Here's how the part is built. I have some questions about the finished solid (model axes, mm). Give positions to 0.01 mm unless a question says otherwise; leave off trailing zeros. Loops run counter-clockwise (first coordinate to the right, second up) from the corner with the lowest first, then second, coordinate; pieces in that order, holes last. Notation, with made-up numbers: (-40, -34) -> (9, -34) arc R27 cw to (9, -5) -> close; hole circle Ø9 at (19.5, 77.25). An arc over 180 degrees is marked (long way). Answer in a Markdown table with one row per item. Add a question column.
Item 1: If we section it at A-A (y = 663): Write out the boundary of the cut face in (x, z).
Item 2: If I drill on line 1 (X direction, y = 740.5, z = -6); line 2 (X direction, y = 880, z = 0); line 3 (X direction, y = 1176, z = 1), over which ranges is the centre line in solid material (lowest first)?
Item 3: For P1, Ø3, axis at x = 0.5, y = 414.5, coming from the -Z side; P2, Ø5, axis at y = 936, z = -1.5, coming from the +X side; P3, Ø8, axis at y = 772.5, z = -0.5, coming from the -X side; P4, Ø5.5, axis at x = 0, z = 0, coming from the -Y side, each with a flat end and sliding along its axis, tell me the tip position at first contact or that it passes through.
```python
from build123d import *

# Parameters (mm, degrees)
BOSS_EXTRU_2_DEPTH      = 1300
ESQUISSE5_R             = 3
ENL_V_MAT_EXTRU_1_DEPTH = 1301.389364767


with BuildPart() as part:
    # Esquisse4 → Boss.-Extru.2 (new body)
    with BuildSketch(Plane(origin=(0, 0, 0), x_dir=(1, 0, 0), z_dir=(0, 1, 0))):
        with BuildLine():
            Line((-17.5, 22.5), (-5, 22.5))
            ThreePointArc((-5, 22.5), (-7.5, 20), (-5, 17.5))
            Line((-5, 17.5), (5, 17.5))
            ThreePointArc((5, 17.5), (7.5, 20), (5, 22.5))
            Line((5, 22.5), (17.5, 22.5))
            ThreePointArc((17.5, 22.5), (21.035534799, 21.035533013), (22.5, 17.499997475))
            Line((22.5, 17.499997475), (22.5, 4.999997475))
            ThreePointArc((22.5, 4.999997475), (20, 7.499997475), (17.5, 4.999997475))
            Line((17.5, 4.999997475), (17.5, -5.000002525))
            ThreePointArc((17.5, -5.000002525), (20, -7.500002525), (22.5, -5.000002525))
            Line((22.5, -5.000002525), (22.5, -17.500002525))
            ThreePointArc((22.5, -17.500002525), (21.035533013, -21.035534799), (17.5, -22.5))
            Line((17.5, -22.5), (5, -22.5))
            ThreePointArc((5, -22.5), (7.5, -20), (5, -17.5))
            Line((5, -17.5), (-5, -17.5))
            ThreePointArc((-5, -17.5), (-7.5, -20), (-5, -22.5))
            Line((-5, -22.5), (-17.5, -22.5))
            ThreePointArc((-17.5, -22.5), (-21.035533906, -21.035533906), (-22.5, -17.5))
            Line((-22.5, -17.5), (-22.5, -5))
            ThreePointArc((-22.5, -5), (-20, -7.5), (-17.5, -5))
            Line((-17.5, -5), (-17.5, 5))
            ThreePointArc((-17.5, 5), (-20, 7.5), (-22.5, 5))
            Line((-22.5, 5), (-22.5, 17.5))
            ThreePointArc((-22.5, 17.5), (-21.035533906, 21.035533906), (-17.5, 22.5))
        make_face()
    extrude(amount=BOSS_EXTRU_2_DEPTH)

    # Esquisse5 → Enlèv. mat.-Extru.1 (cut, through all)
    with BuildSketch(Plane.XZ):
        with Locations(Location((0, 0, 0), (0, 0, 270))):
            Circle(ESQUISSE5_R)
    extrude(amount=-ENL_V_MAT_EXTRU_1_DEPTH, mode=Mode.SUBTRACT)


solid = part.part
```
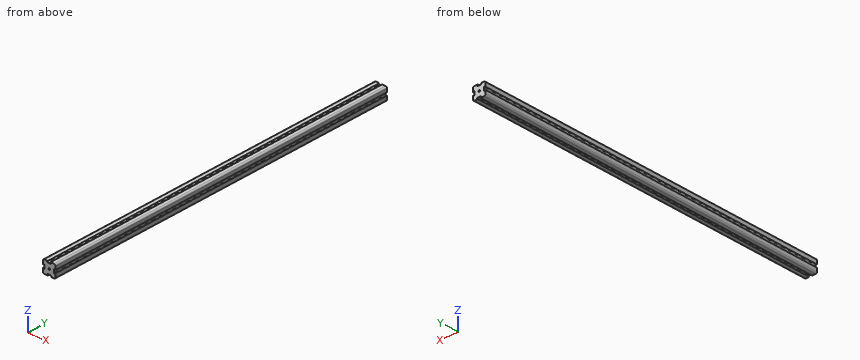
Recorded:
| question | item | result |
|---|---|---|
| 1 | outline | (-22.5, -17.5) arc R5 ccw to (-17.5, -22.5) -> (-5, -22.5) arc R2.5 cw to (-5, -17.5) -> (5, -17.5) arc R2.5 cw to (5, -22.5) -> (17.5, -22.5) arc R5 ccw to (22.5, -17.5) -> (22.5, -5) arc R2.5 cw to (17.5, -5) -> (17.5, 5) arc R2.5 cw to (22.5, 5) -> (22.5, 17.5) arc R5 ccw to (17.5, 22.5) -> (5, 22.5) arc R2.5 cw to (5, 17.5) -> (-5, 17.5) arc R2.5 cw to (-5, 22.5) -> (-17.5, 22.5) arc R5 ccw to (-22.5, 17.5) -> (-22.5, 5) arc R2.5 cw to (-17.5, 5) -> (-17.5, -5) arc R2.5 cw to (-22.5, -5) -> close; hole circle Ø6 at (0, 0) |
| 2 | line 1 | x = -22.5 to -22.29, -17.71 to 17.71, 22.29 to 22.5 |
| 2 | line 2 | x = -17.5 to -3, 3 to 17.5 |
| 2 | line 3 | x = -17.5 to -2.83, 2.83 to 17.5 |
| 3 | P1 | stops at z = -17.5 |
| 3 | P2 | stops at x = 17.5 |
| 3 | P3 | stops at x = -17.5 |
| 3 | P4 | passes through |
